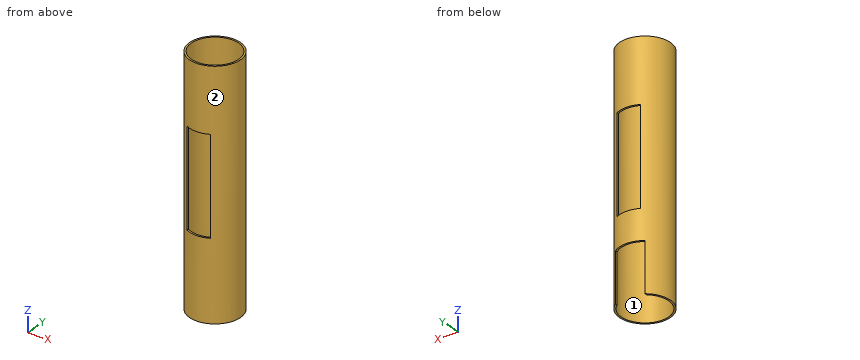
from build123d import *

# Parameters (mm, degrees)
SKETCH1_R               = 31.75
SKETCH1_R_2             = 29.5
BOSS_EXTRUDE1_DEPTH     = 300
CUT_EXTRUDE1_REACH      = 305.342
CUT_EXTRUDE1_END_RADIUS = 31.75
SKETCH2_W               = 37
SKETCH2_H               = 62
CUT_EXTRUDE2_DEPTH      = 304.341597873
CUT_EXTRUDE2_DEPTH_BACK = 304.341597873
SKETCH4_W               = 29.5
SKETCH4_H               = 121


with BuildPart() as part:
    # Sketch1 → Boss-Extrude1 (new body)
    with BuildSketch(Plane.XY):
        Circle(SKETCH1_R)
        Circle(SKETCH1_R_2, mode=Mode.SUBTRACT)
    extrude(amount=BOSS_EXTRUDE1_DEPTH)

    # Cut-Extrude1: up to this cylinder (the profile starts inside it)
    cut_extrude1_end = Plane(origin=(0, 0, 31), z_dir=(0, 0, -1)) * Cylinder(CUT_EXTRUDE1_END_RADIUS, 675.184, mode=Mode.PRIVATE)
    # Sketch2 → Cut-Extrude1 (cut, up to the surface)
    with BuildSketch(Plane(origin=(0, 0, 0), x_dir=(1, 0, 0), z_dir=(0, 1, 0)), mode=Mode.PRIVATE) as cut_extrude1_sk1:
        with Locations((0, -31)):
            Rectangle(SKETCH2_W, SKETCH2_H)
    cut_extrude1_tool1 = extrude(cut_extrude1_sk1.sketch, amount=CUT_EXTRUDE1_REACH, mode=Mode.PRIVATE) & cut_extrude1_end
    add(cut_extrude1_tool1.solids().sort_by_distance((0, 0, 31))[0], mode=Mode.SUBTRACT)

    # Sketch4 → Cut-Extrude2 (cut, two sides: drawn at the far end of the back side and taken through both)
    with BuildSketch(Plane(origin=(0, 0, 0), x_dir=(1, 0, 0), z_dir=(0, 1, 0)).offset(-CUT_EXTRUDE2_DEPTH_BACK)):
        with Locations((0, -160)):
            Rectangle(SKETCH4_W, SKETCH4_H)
    extrude(amount=CUT_EXTRUDE2_DEPTH + CUT_EXTRUDE2_DEPTH_BACK, mode=Mode.SUBTRACT)


solid = part.part
Input: part model. Units: mm. Frame: model coordinates. Face numbers are marked on the shaded views. Round coordinates to 2 decimals unless told otherwise and drop trailing zeros. Write each loop counter-clockwise with the first axis right and the second up, starting at its lowest first coordinate (ties: lowest second). Pieces come first, ordered by that corner, then holes.
1) Cut plane C-C (z = 154.5). Return the cut outline in (x, y), then the cut area to 3 significant figures.
2) Cut plane B-B (x = 0). Return the cut outline in (y, z), then the cut area to 3 significant figures.
3) Draft query along X for the marked faces 1 and 2. Return one class per face: pulls with the +X half, pulls with the -X half, needs draft (parallel to the pull), parting line crosses it, or undercut.
4) Contact query for flat-ended pins moving along their axis: P1, Ø1.5, axis at y = -25.5, z = 146, coming from the -X side; P2, Ø5, axis at x = -4, y = 29, coming from the -Z side; P3, Ø12, axis at x = -13, y = -23, coming from the +Z side; P4, Ø0.8, axis at y = 27, z = 177.5, coming from the +X side (3 decimals). Output: stop coordinate, or through.
5) Cut plane D-D (z = 246). Return the cut outline in (x, y), then the cut area to 3 significant figures.
6) Cut plane A-A (y = 0). Return the cut outline in (x, z).
7) Ray query, L1, parallel to X at y = 0, z = 95; L2, parallel to X at y = 4, z = 173. Return the intervals inside material, ascending.
Geometry says:
1. outline: (-14.75, -28.12) - (-14.75, -25.55) arc R29.5 cw to (-14.75, 25.55) - (-14.75, 28.12) arc R31.75 ccw to start; (14.75, -28.12) arc R31.75 ccw to (14.75, 28.12) - (14.75, 25.55) arc R29.5 cw to (14.75, -25.55) - close
1. area: 294 mm2
2. outline: (-31.75, 0) - (-29.5, 0) - (-29.5, 99.5) - (-31.75, 99.5) - close; (-31.75, 220.5) - (-29.5, 220.5) - (-29.5, 300) - (-31.75, 300) - close; (29.5, 62) - (31.75, 62) - (31.75, 99.5) - (29.5, 99.5) - close; (29.5, 220.5) - (31.75, 220.5) - (31.75, 300) - (29.5, 300) - close
2. area: 666 mm2
3. face 1: undercut
3. face 2: parting line crosses it
4. P1: stops at x = -19.89
4. P2: stops at z = 62
4. P3: stops at z = 300
4. P4: stops at x = 17.335
5. outline: circle Ø63.5 at (0, 0); hole circle Ø59 at (0, 0)
5. area: 433 mm2
6. outline: (-31.75, 0) - (-29.5, 0) - (-29.5, 300) - (-31.75, 300) - close; (29.5, 0) - (31.75, 0) - (31.75, 300) - (29.5, 300) - close
7. L1: x = -31.75 to -29.5, 29.5 to 31.75
7. L2: x = -31.5 to -29.23, 29.23 to 31.5
